Autodesk Inventor part; units mm, degrees
ref_plane "YZ Plane" through (0, 0, 0) normal (1, 0, 0) x (0, 1, 0)
ref_plane "XZ Plane" through (0, 0, 0) normal (0, 1, 0) x (-1, 0, 0)
ref_plane "XY Plane" through (0, 0, 0) normal (0, 0, 1) x (1, 0, 0)
sketch "Sketch1" plane through (0, 0, 0) normal (0, 1, 0) x (-1, 0, 0)
  line L0 (15, 7.5) -> (-15, 7.5)
  line L1 (-15, 7.5) -> (-15, -7.5)
  line L2 (-15, -7.5) -> (15, -7.5)
  line L3 (15, -7.5) -> (15, 7.5)
  line L4 (15, 7.5) -> (-15, -7.5) construction
  line L5 (-15, 7.5) -> (15, -7.5) construction
  line L6 (15, 7.5) -> (13, 7.5)
  line L7 (13, 7.5) -> (13, -7.5)
  line L8 (13, -7.5) -> (15, -7.5)
  line L9 (15, -7.5) -> (15, 7.5)
  circle A0 centre (6, 0) radius 1.5
  circle A1 centre (6, 0) radius 2.75
  line L10 (0, 7.5) -> (0, -7.5) construction
  circle A2 centre (-6, 0) radius 1.5
  circle A3 centre (-6, 0) radius 2.75
  point P0 (0, 0)
  dimension "d0" = 30
  dimension "d1" = 15
  dimension "d2" = 2
  dimension "d3" = 3
  dimension "d4" = 5.5
  dimension "d5" = 6
extrude "Extrusion1" add sketch "Sketch1" along normal blind 2 contours L7 L2 L1 L0
extrude "Extrusion2" add sketch "Sketch1" along normal blind 29 contours L3 L2 L7 L0
extrude "Extrusion3" add sketch "Sketch1" along normal blind 1 contours A1 | A3
sketch "Sketch2" plane through (-13, 2, -7.5) normal (1, 0, 0) x (0, 0, -1)
  line L0 (0, 0) -> (0, 27)
  line L1 (0, 0) -> (-15, 0)
  circle A0 centre (0, 12.25) radius 12.25
  point P0 (-7.5, -2)
  point P1 (0, 13.5)
  point P2 (0, 24.5)
  dimension "d16" = 24.5
  dimension "d17" = 12.25
extrude "Extrusion4" cut sketch "Sketch2" against normal blind 2 contours A0 L0 picked at (-3.685, 9.0749)
sketch "Sketch3" plane through (-13, 2, 7.5) normal (1, 0, 0) x (0, 0, -1)
  line L0 (0, 27) -> (15, 27)
  line L1 (15, 27) -> (0, 27)
  line L2 (0, 0) -> (0, 27)
  line L3 (0, 27) -> (0, 0)
  line L4 (0, 0) -> (15, 0)
  arc A0 (15, 24.5) -> (15, 0) centre (15, 12.25) ccw
  arc A1 (2.75, 12.25) -> (15, 24.5) centre (15, 12.25) ccw
  line L5 (15, 27) -> (15, 24.5)
  line L6 (15, 0) -> (15, 24.5)
  point P0 (7.5, -2)
extrude "Extrusion5" add sketch "Sketch3" along normal blind 3 contours L0 L5 A0 L4 L2
properties part number "Bracket Motor JGA Kiri_3DPrint"
Design review of the part built by this model. Coordinates are the model's own, in mm. A direction names the side the tool comes from. Round coordinates to 2 decimals unless told otherwise and drop trailing zeros. Write each loop counter-clockwise with the first axis right and the second up, starting at its lowest first coordinate (ties: lowest second). Pieces come first, ordered by that corner, then holes. Notation, with made-up numbers: (34.25, 41) -> (81.25, 41) arc R24 ccw to (81.25, 63) -> close; hole circle Ø10 at (-39, -34.5). An arc over 180 degrees is marked (long way). One line per question, with ' | ' between items.
(1) Machinability: for faces 1 (the flat face through (-10, 19, 5)), 2 (the flat face through (4.8, 1, -1.2)), 3 (the flat face through (15, 1, 0)), which of the approach directions +Z, -Z, +X, -X, +Y, -Y give a long, thin tool a straight path to every point of the face, cutting with its end or side? Answer none if there is none.
Result sheet:
face 1: +Z, -Z, +X, +Y | face 2: +Y | face 3: +Z, -Z, +X, +Y, -Y
(2) Wall thickness on line 1 (Z direction, x = 6, y = 1.85); line 2 (X direction, y = 16.5, z = 5.5); line 3 (Y direction, x = 1, z = 5): over which ranges is each line inside the solid? List them lowest first. Write a range as [from, to].
Result sheet:
line 1: [-7.5, -2.75], [2.75, 7.5] | line 2: [-15, -10] | line 3: [0, 2]
(3) Take a section at C-C, the plane x = 12.5. State the section outline as (y, z) points, and give its area (3 significant figures).
Result sheet:
outline: (0, -7.5) -> (2, -7.5) -> (2, 7.5) -> (0, 7.5) -> close | area: 30.0 mm2
(4) Take a section at B-B, the plane z = 4. State the section outline as (x, y) points, and give its area (3 significant figures).
Result sheet:
outline: (-15, 0) -> (15, 0) -> (15, 2) -> (-10, 2) -> (-10, 10.03) -> (-15, 10.03) -> close; (-15, 18.47) -> (-10, 18.47) -> (-10, 29) -> (-15, 29) -> close | area: 153 mm2
(5) Insertion check: P1, Ø1.6, axis at x = -6, z = -1.5, coming from the +Y side; P2, Ø4.5, axis at x = -6, z = 0, coming from the -Y side; P3, Ø4.5, axis at x = 6.5, z = -3, coming from the +Y side; P4, Ø5, axis at y = 9.5, z = 4, coming from the +X side. Each pin has a flat end and moves straight along its axis. Give the tip position at first contact, or say it passes through.
Result sheet:
P1: y = 1 | P2: y = 0 | P3: y = 2 | P4: x = -10
(6) Take a section at D-D, the plane y = 14.25. State the section outline as (x, z) points.
Result sheet:
outline: (-15, 4.75) -> (-10, 4.75) -> (-10, 7.5) -> (-15, 7.5) -> close
(7) Take a section at A-A, the plane x = -6. State the section outline as (y, z) points.
Result sheet:
outline: (0, -7.5) -> (2, -7.5) -> (2, -2.75) -> (1, -2.75) -> (1, -1.5) -> (0, -1.5) -> close; (0, 1.5) -> (1, 1.5) -> (1, 2.75) -> (2, 2.75) -> (2, 7.5) -> (0, 7.5) -> close
(8) Draft analysis for pull direction Z (two halves, no side actions). For faces 4 (the flat face through (3, 2, 0)), 5 (the cylindrical face through (3.46, 1.49, 1.05)), 6 (the cylindrical face through (-12.465, 14.519, 4.747)), state which applies: released by +Z, released by -Z, zero draft, split by the parting line, or undercut.
Result sheet:
face 4: zero draft | face 5: undercut | face 6: released by -Z
